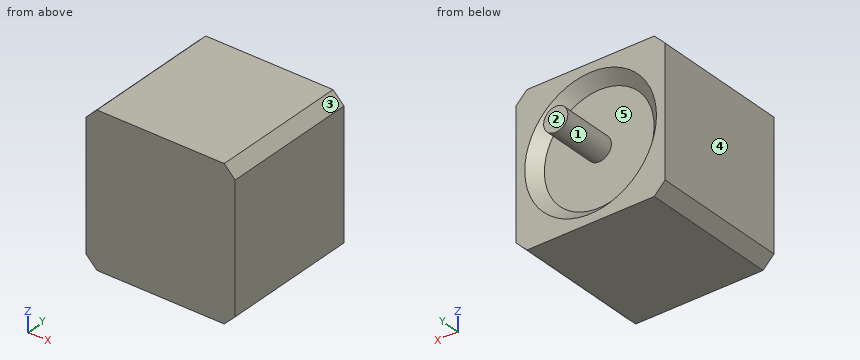
```python
from build123d import *

# Parameters (mm, degrees)
SKETCH1_W           = 86.36
SKETCH1_H           = 86.36
BOSS_EXTRUDE1_DEPTH = 80.01
SKETCH2_R           = 31.75
CUT_EXTRUDE1_DEPTH  = 6.35
CHAMFER1_SIZE       = 6.35
SKETCH3_R           = 6.99897
BOSS_EXTRUDE2_DEPTH = 32.004
CHAMFER2_SIZE       = 6.35


with BuildPart() as part:
    # Sketch1 → Boss-Extrude1 (new body)
    with BuildSketch(Plane(origin=(0, 0, 0), x_dir=(1, 0, 0), z_dir=(0, 1, 0))):
        Rectangle(SKETCH1_W, SKETCH1_H)
    extrude(amount=BOSS_EXTRUDE1_DEPTH)

    # Sketch2 → Cut-Extrude1 (cut)
    with BuildSketch(Plane(origin=(0, 80.01, 0), x_dir=(1, 0, 0), z_dir=(0, 1, 0))):
        with Locations(Location((0, 0, 0), (0, 0, 270))):
            Circle(SKETCH2_R)
    extrude(amount=-CUT_EXTRUDE1_DEPTH, mode=Mode.SUBTRACT)

    # Chamfer1
    chamfer1_edges = [part.edges().sort_by_distance(p)[0] for p in [
        (43.18, 40.005, 43.18),
        (-43.18, 40.005, 43.18),
        (-43.18, 40.005, -43.18),
        (43.18, 40.005, -43.18),
    ]]
    chamfer(chamfer1_edges, length=CHAMFER1_SIZE)

    # Sketch3 → Boss-Extrude2 (add)
    with BuildSketch(Plane(origin=(0, 73.66, 0), x_dir=(1, 0, 0), z_dir=(0, 1, 0))):
        with Locations(Location((0, 0, 0), (0, 0, 270))):
            Circle(SKETCH3_R)
    extrude(amount=BOSS_EXTRUDE2_DEPTH)

    # Chamfer2
    chamfer2_edges = [part.edges().sort_by_distance(p)[0] for p in [
        (0, 80.01, -31.75),
    ]]
    chamfer(chamfer2_edges, length=CHAMFER2_SIZE - 0.0001)  # a hair under: the kernel refuses the full size


solid = part.part
```
The model under review builds one solid part; all positions refer to its coordinate system, in mm. Face numbers are marked on the shaded views. A direction names the side the tool comes from. Coordinates: 2 decimals unless noted, no trailing zeros. Write each loop counter-clockwise with the first axis right and the second up, starting at its lowest first coordinate (ties: lowest second). Pieces come first, ordered by that corner, then holes. Notation, with made-up numbers: (34, 41) -> (48, 41) arc R13 ccw to (48, 53) -> close; hole circle Ø9 at (-12.5, 53). An arc over 180 degrees is marked (long way). One line per item, written item: value. Start each with the question number.
Q1. Add section A-A, the plane y = 76.5. Give the boundary of the cut face in (x, z), then the cut area to 3 significant figures.
Q2. To check wall thickness, follow probe 1 along X at (y, z) = (73.75, 0); probe 2 along Y at (x, z) = (39.5, -6.5); probe 3 along Y at (x, z) = (30.5, -6). State the ranges of each line that lie inside material, in increasing order.
Q3. Clearance check with flat-ended pins moving along their axes: P1, Ø2, axis at x = 34.5, z = -1, coming from the +Y side; P2, Ø5, axis at x = -9.5, z = 17, coming from the +Y side. State where each tip first meets the part, or that it passes through.
Q4. For the marked faces 1 and 2, list the 3-axis set-ups (+Z, -Z, +X, -X, +Y, -Y) from which the entire face can be reached by the end or side of a thin tool; tool diameter is ignored.
Q5. The part is to be moulded in two halves that separate along X. For the marked faces 3, 4 and 5, say which applies: +X half, -X half, draft (parallel to the pull), parting line (faces both ways), or undercut.
Response:
1. outline: (-43.18, -36.83) -> (-36.83, -43.18) -> (36.83, -43.18) -> (43.18, -36.83) -> (43.18, 36.83) -> (36.83, 43.18) -> (-36.83, 43.18) -> (-43.18, 36.83) -> close; circle Ø14 at (0, 0); hole circle Ø69.18 at (0, 0)
1. area: 3,770 mm²
2. probe 1: -43.18 to -31.84, -7 to 7, 31.84 to 43.18
2. probe 2: 0 to 80.01
2. probe 3: 0 to 73.66
3. P1: y = 77.42
3. P2: y = 73.66
4. face 1: +Y
4. face 2: +Z, -Z, +X, -X, +Y
5. face 3: +X half
5. face 4: -X half
5. face 5: undercut
